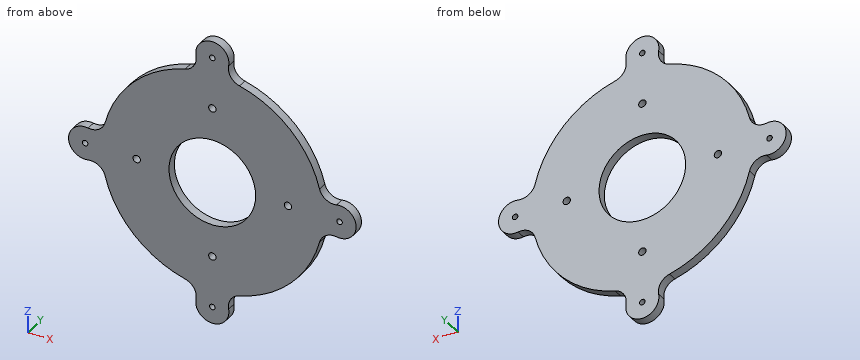
```python
from build123d import *

# Parameters (mm, degrees)
SKETCH1_R           = 23.5
SKETCH1_R_2         = 1.5
SKETCH1_R_3         = 2
BOSS_EXTRUDE1_DEPTH = 5


with BuildPart() as part:
    # Sketch1 → Boss-Extrude1 (new body)
    with BuildSketch(Plane(origin=(0, 0, 0), x_dir=(1, 0, 0), z_dir=(0, 1, 0))):
        with BuildLine():
            ThreePointArc((58.158567775, 14.750626914), (42.426406871, 42.426406871), (14.750626914, 58.158567775))
            ThreePointArc((14.750626914, 58.158567775), (9.981753959, 61.596635254), (8.850376149, 67.3657289))
            ThreePointArc((8.850376149, 67.3657289), (0, 78), (-8.850376149, 67.3657289))
            ThreePointArc((-8.850376149, 67.3657289), (-9.981753959, 61.596635254), (-14.750626914, 58.158567775))
            ThreePointArc((-14.750626914, 58.158567775), (-42.426406871, 42.426406871), (-58.158567775, 14.750626914))
            ThreePointArc((-58.158567775, 14.750626914), (-61.596635254, 9.981753959), (-67.3657289, 8.850376149))
            ThreePointArc((-67.3657289, 8.850376149), (-78, 0), (-67.3657289, -8.850376149))
            ThreePointArc((-67.3657289, -8.850376149), (-61.596635254, -9.981753959), (-58.158567775, -14.750626914))
            ThreePointArc((-58.158567775, -14.750626914), (-42.426406871, -42.426406871), (-14.750626914, -58.158567775))
            ThreePointArc((-14.750626914, -58.158567775), (-9.981753959, -61.596635254), (-8.850376149, -67.3657289))
            ThreePointArc((-8.850376149, -67.3657289), (0, -78), (8.850376149, -67.3657289))
            ThreePointArc((8.850376149, -67.3657289), (9.981753959, -61.596635254), (14.750626914, -58.158567775))
            ThreePointArc((14.750626914, -58.158567775), (42.426406871, -42.426406871), (58.158567775, -14.750626914))
            ThreePointArc((58.158567775, -14.750626914), (61.596635254, -9.981753959), (67.3657289, -8.850376149))
            ThreePointArc((67.3657289, -8.850376149), (78, 0), (67.3657289, 8.850376149))
            ThreePointArc((67.3657289, 8.850376149), (61.596635254, 9.981753959), (58.158567775, 14.750626914))
        make_face()
        Circle(SKETCH1_R, mode=Mode.SUBTRACT)
        with Locations((69, 0)):
            Circle(SKETCH1_R_2, mode=Mode.SUBTRACT)
        with Locations((41.01219331, 0)):
            Circle(SKETCH1_R_3, mode=Mode.SUBTRACT)
        with Locations((0, 41.01219331)):
            Circle(SKETCH1_R_3, mode=Mode.SUBTRACT)
        with Locations((-41.01219331, 0)):
            Circle(SKETCH1_R_3, mode=Mode.SUBTRACT)
        with Locations((0, -41.01219331)):
            Circle(SKETCH1_R_3, mode=Mode.SUBTRACT)
        with Locations((0, 69)):
            Circle(SKETCH1_R_2, mode=Mode.SUBTRACT)
        with Locations((0, -69)):
            Circle(SKETCH1_R_2, mode=Mode.SUBTRACT)
        with Locations((-69, 0)):
            Circle(SKETCH1_R_2, mode=Mode.SUBTRACT)
    extrude(amount=BOSS_EXTRUDE1_DEPTH)


solid = part.part
```
CAD build for the part. Positions are in the model's coordinates, mm. Round coordinates to 2 decimals unless told otherwise and drop trailing zeros. Write each loop counter-clockwise with the first axis right and the second up, starting at its lowest first coordinate (ties: lowest second). Pieces come first, ordered by that corner, then holes.
Item 1: Band-saw the part on B-B on x = 35. Write the cut outline in (y, z).
Filled in:
outline: (0, -48.73) - (5, -48.73) - (5, 48.73) - (0, 48.73) - close
Item 2: Drill centre lines: L1, parallel to X at y = 1.7, z = 0; L2, parallel to Z at x = -69, y = 1.65. Where is each one in solid material? Low to high.
Filled in:
L1: x = -78 to -70.5, -67.5 to -43.01, -39.01 to -23.5, 23.5 to 39.01, 43.01 to 67.5, 70.5 to 78
L2: z = -9 to -1.5, 1.5 to 9
Item 3: Drop flat-ended pins along their axis: pin 1 Ø2.5 at (x, z) = (0, -69) entering from -Y; pin 2 Ø1 at (y, z) = (4.5, -26.5) entering from +X. Give the stop position or say it passes through.
Filled in:
pin 1: passes through
pin 2: stops at x = 54.07
Item 4: Band-saw the part on A-A on y = 3.35. Give the number of separate pieces and of enclosed holes in the cut face, then the cut area to 3 significant figures.
Filled in:
separate pieces: 1
enclosed holes: 9
area: 10,700 mm2
Item 5: Band-saw the part on C-C on z = -29. Write the cut outline in (x, y), then the cut area to 3 significant figures.
Filled in:
outline: (-52.53, 0) - (52.53, 0) - (52.53, 5) - (-52.53, 5) - close
area: 525 mm2
